Can you work these out from the model? Positions are in its coordinate system, mm. Round coordinates to 2 decimals unless told otherwise and drop trailing zeros. Order: outer loops, then holes, each group sorted by start corner. A loop starts at its lowest first (then second) coordinate and runs counter-clockwise, first axis right, second up. Notation, with made-up numbers: M 19,-27 L 56,-27 A32 ccw 56,6 Z; hole C 26,70 d1. An arc over 180 degrees is marked long. Answer as a JSON object with one key per item and string values. Group by question number.
from build123d import *

# Parameters (mm, degrees)
F1_DEPTH = 495


with BuildPart() as f1:
    # F0 (on Front) → F1 (new body, symmetric)
    with BuildSketch(Plane.XZ):
        with BuildLine():
            Line((-20, -2.5), (20, -2.5))
            Line((20, -2.5), (20, 2.5))
            Line((20, 2.5), (8.9, 2.5))
            Line((8.9, 2.5), (8.9, 9.2))
            Line((8.9, 9.2), (7.68, 9.2))
            Line((7.68, 9.2), (4.000485, 15.572077))
            ThreePointArc((4.000485, 15.572077), (0, 30.5), (-4.000485, 15.572077))
            Line((-4.000485, 15.572077), (-7.68, 9.2))
            Line((-7.68, 9.2), (-8.9, 9.2))
            Line((-8.9, 9.2), (-8.9, 2.5))
            Line((-8.9, 2.5), (-20, 2.5))
            Line((-20, 2.5), (-20, -2.5))
        make_face()
    extrude(amount=F1_DEPTH, both=True)


solid = f1.part
Item 1: Suppose I cut it at B-B, the plane z = 22.5. Write out the boundary of the cut face in (x, y), and give its area (3 significant figures).
Item 2: I'm going to push flat-ended pins straight in: pin 1 Ø5.5 at (x, y) = (12, -212) entering from +Z; pin 2 Ø2 at (y, z) = (-184, 5) entering from +X; pin 3 Ø0.6 at (x, y) = (8.5, -113.5) entering from +Z; pin 4 Ø6 at (x, z) = (-9.5, 15.5) entering from -Y. Where does each tip first touch, or does it pass through?
Item 3: If we mould it in two halves opening along Z, with no side actions, what happens to faces 1 (the face through (0, -7, -2.5)), 2 (the face through (0.293, -6.93, 30.495)), 3 (the face through (0, -495, 11))? For each: +Z half, -Z half, draft (parallel to the pull), parting line (faces both ways), or undercut.
Item 4: I need wall thicknesses on line 1 (X direction, y = -421.5, z = 6); line 2 (Z direction, x = -12.5, y = -265); line 3 (Z direction, x = 1, y = 143). Which ranges of each line are inside material? Lowest first, please.
Item 5: Suppose I cut it at A-A, the plane y = -343.5. Write out the boundary of the cut face in (x, z).
Computed:
{
 "1": {"outline": "M -8,-495 L 8,-495 L 8,495 L -8,495 Z", "area": "15,800 mm^2"},
 "2": {"pin 1": "stops at z = 2.5", "pin 2": "stops at x = 8.9", "pin 3": "stops at z = 9.2", "pin 4": "passes through"},
 "3": {"face 1": "-Z half", "face 2": "undercut", "face 3": "draft"},
 "4": {"line 1": "x = -8.9 to 8.9", "line 2": "z = -2.5 to 2.5", "line 3": "z = -2.5 to 30.44"},
 "5": {"outline": "M -20,-2.5 L 20,-2.5 L 20,2.5 L 8.9,2.5 L 8.9,9.2 L 7.68,9.2 L 4,15.57 A8 ccw long -4,15.57 L -7.68,9.2 L -8.9,9.2 L -8.9,2.5 L -20,2.5 Z"}
}
